Model file for the job. Use its own axes, mm. Face numbers are marked on the shaded views. A direction names the side the tool comes from. Round coordinates to 2 decimals unless told otherwise and drop trailing zeros. Order: outer loops, then holes, each group sorted by start corner. A loop starts at its lowest first (then second) coordinate and runs counter-clockwise, first axis right, second up. Notation, with made-up numbers: (82.5, 81) - (117.5, 81) arc R12 ccw to (117.5, 91) - close; hole circle Ø7 at (70, 25). An arc over 180 degrees is marked (long way). Put each result on its own line as item: value. Start each with the question number.
Item 1: Which spindle directions (+Z, -Z, +X, -X, +Y, -Y) get a long thin tool onto all of the face, cutting with end or side? Do the marked faces 1, 2, 3 and 4. Say none if no direction does.
Item 2: Saw through at B-B on y = -21. List the corners of the cut face in (x, z) (3 decimals).
Item 3: Mould opens along Z. For the marked faces 5, 6, 7 and 8 say: pulls with the +Z half, pulls with the -Z half, needs draft (parallel to the pull), parting line crosses it, or undercut.
Item 4: Saw through at C-C on x = -73. List the corners of the cut face in (y, z), plus the area to 3 significant figures.
Item 5: Pin check, flat tips, straight feed: pin 1 Ø7.5 at (x, y) = (24.5, 1) entering from -Z; pin 2 Ø12.5 at (y, z) = (-0.5, -10.5) entering from +X; pin 3 Ø16 at (x, y) = (17.5, -4.5) entering from +Z; pin 4 Ø5.5 at (x, y) = (38.1, -2.82) entering from -Z. Stop position of each tip, or through.
Item 6: Saw through at A-A on x = 22.5. List the corners of the cut face in (y, z).
Item 7: Probe probe 1 along Z at (x, y) = (20, -0.5); probe 2 along Z at (x, y) = (-38, 7.5); probe 3 along Y at (x, z) = (12.7, -21.4). List the from-to ranges inside material, lowest first.
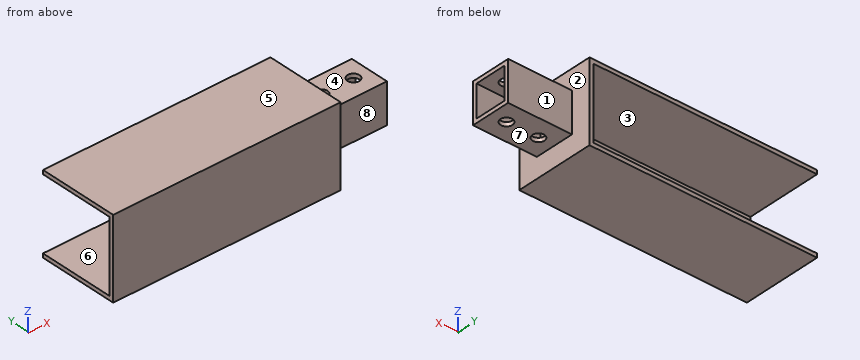
```python
from build123d import *

# Parameters (mm, degrees)
SKETCH1_W                       = 31.75
SKETCH1_H                       = 31.75
SKETCH1_W_2                     = 25.4
SKETCH1_H_2                     = 25.4
BOSS_EXTRUDE1_DEPTH             = 50.8
SKETCH2_W                       = 63.5
SKETCH2_H                       = 63.5
BOSS_EXTRUDE2_DEPTH             = 3.175
F_97_0_375_DIAMETER_HOLE1_D     = 9.525
F_97_0_375_DIAMETER_HOLE1_DEPTH = 76.2
BOSS_EXTRUDE3_DEPTH             = 177.8


with BuildPart() as part:
    # Sketch1 → Boss-Extrude1 (new body)
    with BuildSketch(Plane.YZ):
        with Locations((-2.823153034, -6.41701847)):
            Rectangle(SKETCH1_W, SKETCH1_H)
        with Locations((-2.823153034, -6.41701847)):
            Rectangle(SKETCH1_W_2, SKETCH1_H_2, mode=Mode.SUBTRACT)
    extrude(amount=BOSS_EXTRUDE1_DEPTH)

    # Sketch2 → Boss-Extrude2 (add)
    with BuildSketch(Plane(origin=(0, 0, 0), x_dir=(0, -1, 0), z_dir=(-1, 0, 0))):
        with Locations((2.823153034, -6.41701847)):
            Rectangle(SKETCH2_W, SKETCH2_H)
    extrude(amount=BOSS_EXTRUDE2_DEPTH)

    # #97 (0.375) Diameter Hole1
    with Locations(Plane.XY.offset(9.45798153)):
        with Locations((38.1, -2.823153034), (12.7, -2.823153034)):
            Hole(F_97_0_375_DIAMETER_HOLE1_D / 2, depth=F_97_0_375_DIAMETER_HOLE1_DEPTH)

    # Sketch7 → Boss-Extrude3 (add)
    with BuildSketch(Plane.ZY.offset(3.175)):
        Polygon((-38.16701847, 28.926846966), (-34.99201847, 28.926846966), (-34.99201847, -31.398153034), (22.15798153, -31.398153034), (22.15798153, 28.926846966), (25.33298153, 28.926846966), (25.33298153, -34.573153034), (-38.16701847, -34.573153034), align=None)
    extrude(amount=BOSS_EXTRUDE3_DEPTH)


solid = part.part
```
Results found:
1. face 1: +Z, -Z, +X, +Y
1. face 2: +X
1. face 3: -X, +Y
1. face 4: +Z, +X, +Y, -Y
2. outline: (-180.975, -38.167) - (0, -38.167) - (0, 25.333) - (-180.975, 25.333) - (-180.975, 22.158) - (-3.175, 22.158) - (-3.175, -34.992) - (-180.975, -34.992) - close
3. face 5: pulls with the +Z half
3. face 6: undercut
3. face 7: pulls with the -Z half
3. face 8: needs draft
4. outline: (-34.57, -38.17) - (28.93, -38.17) - (28.93, -34.99) - (-31.4, -34.99) - (-31.4, 22.16) - (28.93, 22.16) - (28.93, 25.33) - (-34.57, 25.33) - close
4. area: 585 mm²
5. pin 1: stops at z = -22.29
5. pin 2: stops at x = 0
5. pin 3: stops at z = 9.46
5. pin 4: passes through
6. outline: (-18.7, -22.29) - (13.05, -22.29) - (13.05, 9.46) - (-18.7, 9.46) - close; hole (-15.52, -19.12) - (9.88, -19.12) - (9.88, 6.28) - (-15.52, 6.28) - close
7. probe 1: z = -22.29 to -19.12, 6.28 to 9.46
7. probe 2: z = -38.17 to -34.99, 22.16 to 25.33
7. probe 3: y = -18.7 to -7.59, 1.94 to 13.05
